CAD build for the part. Positions are in the model's coordinates, mm. A direction names the side the tool comes from. Give positions to 0.01 mm unless a question says otherwise; leave off trailing zeros. Order: outer loops, then holes, each group sorted by start corner. A loop starts at its lowest first (then second) coordinate and runs counter-clockwise, first axis right, second up. Notation, with made-up numbers: M 35.5,83.5 L 68.5,83.5 A20 ccw 68.5,103.5 Z; hole C 28,85 d9. An arc over 180 degrees is marked long. Put each result on its own line as item: value. Start each with the question number.
1) Tool access for faces 1 (the face through (0, 0, -10)), 2 (the face through (-40, 0, -20.629)): list every direction of +Z, -Z, +X, -X, +Y, -Y with a clear straight run to the whole face (end or side of a thin tool).
2) Cut at C-C (x = -42). Write the cut outline in (y, z).
3) Drill centre lines: line 1 (X direction, y = 0.85, z = -14.25); line 2 (Z direction, x = -44, y = 0.3); line 3 (Z direction, x = -44, y = 0.65). Where is each one in solid material? Low to high. Write a range as [from, to].
4) Cut at D-D (y = 0.35). Write the cut outline in (x, z), and give its area (3 significant figures).
5) Cut at A-A (z = -16). Write the cut outline in (x, y).
6) Cut at B-B (x = -6). Write the cut outline in (y, z), and give its area (3 significant figures).
7) Pin check, flat tips, straight feed: pin 1 (0.9 mm diameter, centred on x = -11.5, y = -0.5, fed in from -Z); pin 2 (0.9 mm diameter, centred on x = -40.5, y = 0.5, fed in from -Z); pin 3 (1.5 mm diameter, centred on x = -22, y = 1, fed in from -Z). Stop position of each tip, or through.
8) Two-plate mould, pull along Z, no slides. Class faces 3 (the face through (-25, 1.944, -6)), 4 (the face through (-45.5, 0.4, -2.2)), 5 (the face through (-15.406, 0, -14)), 6 (the face through (-24.65, 0.42, -23.37)): released by +Z, released by -Z, zero draft, split by the parting line, or undercut.
Autodesk Inventor part; units mm, degrees
ref_plane "YZ Plane" through (0, 0, 0) normal (1, 0, 0) x (0, 1, 0)
ref_plane "XZ Plane" through (0, 0, 0) normal (0, 1, 0) x (-1, 0, 0)
ref_plane "XY Plane" through (0, 0, 0) normal (0, 0, 1) x (1, 0, 0)
sketch "Sketch1" plane through (0, 0, 0) normal (1, 0, 0) x (0, 1, 0)
  line L0 (1.944, 4.8709) -> (-1.056, 4.8709)
  line L1 (-1.056, 4.8709) -> (-1.056, -25.1291)
  line L2 (-1.056, -25.1291) -> (1.944, -25.1291)
  line L3 (1.944, -25.1291) -> (1.944, 4.8709)
  line L4 (-1.056, -25.1291) -> (9.6963, -12.315)
  point P0 (0, 0)
  point P1 (1.944, -21.5539)
  dimension "d0" = 3
  dimension "d1" = 30
  dimension "d2" = 40
extrude "Extrusion1" add sketch "Sketch1" against normal blind 50 contours L3 L4 L1 L0
sketch "Szkic2" plane through (0, -1.056, -25.1291) normal (0, -1, 0) x (1, 0, 0)
  line L0 (0, 30) -> (0, 0)
  line L1 (0, 30) -> (-50, 30)
  line L2 (-50, 0) -> (-50, 30)
  line L3 (0, 0) -> (-50, 0)
  line L4 (-35.094, 16.557) -> (-35.094, 5.254)
  line L5 (-45, 5) -> (-35.348, 5)
  line L6 (-45, 5) -> (-45, 16.43)
  line L7 (-44.873, 16.557) -> (-35.094, 16.557)
  circle A0 centre (-39.92, 11.35) radius 1
  line L8 (-25, 0) -> (-25, 30)
  line L9 (-35.094, 5.254) -> (-35.348, 5)
  line L10 (-45.5, 16.43) -> (-45.5, 4.5)
  line L11 (-45.5, 4.5) -> (-35.1409, 4.5)
  line L12 (-34.594, 5.0469) -> (-34.594, 17.057)
  line L13 (-34.594, 17.057) -> (-44.873, 17.057)
  line L14 (-35.1409, 4.5) -> (-35.094, 4.5469)
  line L15 (-34.6409, 5) -> (-34.594, 5.0469)
  line L16 (-45.5, 4.5) -> (-34.594, 4.5)
  line L17 (-34.594, 4.5) -> (-34.594, 17.057)
  line L18 (-34.594, 17.057) -> (-45.5, 17.057)
  line L19 (-45.5, 17.057) -> (-45.5, 4.5)
  circle A1 centre (-10.08, 11.35) radius 1
  line L20 (-4.5, 16.43) -> (-4.5, 4.5)
  line L21 (-4.5, 4.5) -> (-14.8591, 4.5)
  line L22 (-15.406, 5.0469) -> (-15.406, 17.057)
  line L23 (-15.406, 17.057) -> (-5.127, 17.057)
  line L24 (-4.5, 4.5) -> (-15.406, 4.5)
  line L25 (-15.406, 4.5) -> (-15.406, 17.057)
  line L26 (-15.406, 17.057) -> (-4.5, 17.057)
  line L27 (-4.5, 17.057) -> (-4.5, 4.5)
  line L28 (0, 4.1492) -> (-50, 4.1492)
  line L29 (-50, 4.1492) -> (-50, 27.66)
  line L30 (-36.5, 27.66) -> (-50, 27.66)
  line L31 (-36.5, 27.66) -> (-36.5, 17.057)
  line L32 (-26.5, 4.66) -> (-36.5, 4.66)
  line L33 (-26.5, 4.66) -> (-26.5, 34.4086)
  line L34 (-23.5, 34.4086) -> (-23.5, 4.66)
  line L35 (-13.5, 4.66) -> (-23.5, 4.66)
  line L36 (-13.5, 4.66) -> (-13.5, 13.5389)
  line L37 (0, 27.66) -> (-13.5, 27.66)
  line L38 (0, 4.1492) -> (0, 27.66)
  line L39 (-50, 4.1492) -> (-44, 4.1492)
  line L40 (-44, 27.66) -> (-50, 27.66)
  line L41 (-50, 27.66) -> (-50, 4.1492)
  line L42 (-50, 27.66) -> (-36.5, 27.66)
  line L43 (-36.5, 27.66) -> (-36.5, 24.66)
  line L44 (-50, 24.66) -> (-50, 27.66)
  circle A2 centre (-10.08, 11.35) radius 1
  circle A3 centre (-39.92, 11.35) radius 1
  line L45 (-6, 27.66) -> (-6, 22.91)
  line L46 (-44, 27.66) -> (-44, 22.91)
  circle A4 centre (-6, 22.91) radius 1.5
  circle A5 centre (-44, 22.91) radius 1.5
  circle A6 centre (-6, 22.91) radius 1.75
  circle A7 centre (-44, 22.91) radius 1.75
  line L47 (-12.975, 17.057) -> (-13.5, 17.057)
  line L48 (-36.5, 17.057) -> (-37.0252, 17.057)
  line L49 (-45.5, 15.557) -> (-45.5, 15.0389)
  line L50 (-37.0252, 13.5389) -> (-36.5, 13.5389)
  line L51 (-36.5, 13.5389) -> (-36.5, 4.66)
  line L52 (-13.5, 13.5389) -> (-12.975, 13.5389)
  line L53 (-4.5, 15.0389) -> (-4.5, 15.557)
  arc A8 (-12, 17.057) -> (-12.975, 16.6969) centre (-12, 15.557) ccw
  line L54 (-12.975, 16.6969) -> (-12.975, 17.057)
  line L55 (-37.0252, 16.697) -> (-37.0252, 17.057)
  arc A9 (-37.0252, 16.697) -> (-38, 17.057) centre (-38, 15.557) ccw
  arc A10 (-44, 17.057) -> (-45.5, 15.557) centre (-44, 15.557) ccw
  arc A11 (-45.5, 15.0389) -> (-44, 13.5389) centre (-44, 15.0389) ccw
  arc A12 (-38, 13.5389) -> (-37.0252, 13.8988) centre (-38, 15.0389) ccw
  line L56 (-37.0252, 13.8988) -> (-37.0252, 13.5389)
  line L57 (-12.975, 13.899) -> (-12.975, 13.5389)
  arc A13 (-12.975, 13.899) -> (-12, 13.5389) centre (-12, 15.0389) ccw
  line L58 (-12, 13.5389) -> (-6, 13.5389)
  arc A14 (-6, 13.5389) -> (-4.5, 15.0389) centre (-6, 15.0389) ccw
  arc A15 (-4.5, 15.557) -> (-6, 17.057) centre (-6, 15.557) ccw
  line L59 (-6, 17.057) -> (-12, 17.057)
  line L60 (-38, 17.057) -> (-44, 17.057)
  line L61 (-44, 13.5389) -> (-38, 13.5389)
  arc A16 (-26.5, 34.4086) -> (-23.5, 34.4086) centre (-25, 35.31) ccw
  line L62 (-13.5, 17.057) -> (-13.5, 27.66)
  point P0 (0, 25.1291)
  point P1 (-45.5, 13.5389)
  point P2 (-4.5, 13.5389)
extrude "Wyciągnięcie proste2" cut sketch "Szkic2" against normal through all contours L35 L36 L52 L57 A13 L58 A14 L20 L21 L24 L25 | L25 L22 L23 L54 A8 A15 L20 A14 L58 A13 L57 L52 L36 L35 | L23 A8 L54 | L32 L51 L50 L56 A12 L61 A11 L10 A10 L13 A9 L55 L12 L17 | L17 L16 L11 L10 A11 L6 L5 L51 L32 | L23 L26 L27 L20 A15 | L5 L6 A11 L61 A12 L56 L50 L51 | L55 A9 L13 | L10 L19 L18 L13 A10 | A0 | A1
sketch "Szkic3" plane through (0, -1.056, -25.1291) normal (0, -1, 0) x (1, 0, 0)
  line L0 (-4.5, 17.057) -> (-4.5, 4.5)
  line L1 (-4.5, 4.5) -> (-15.406, 4.5)
  line L2 (-15.406, 4.5) -> (-15.406, 17.057)
  line L3 (-15.406, 17.057) -> (-4.5, 17.057)
  line L4 (-34.594, 17.057) -> (-34.594, 4.5)
  line L5 (-34.594, 4.5) -> (-45.5, 4.5)
  line L6 (-45.5, 4.5) -> (-45.5, 17.057)
  line L7 (-45.5, 17.057) -> (-34.594, 17.057)
  line L8 (0, 30) -> (0, 0)
  line L9 (0, 30) -> (-50, 30)
  line L10 (-50, 0) -> (-50, 30)
  line L11 (0, 0) -> (-50, 0)
  circle A0 centre (-44, 24.66) radius 1.75
  circle A1 centre (-10.08, 11.35) radius 1
  circle A2 centre (-39.92, 11.35) radius 1
  line L12 (0, 4.1492) -> (-50, 4.1492)
  line L13 (-50, 4.1492) -> (-50, 27.66)
  line L14 (-36.5, 27.66) -> (-50, 27.66)
  line L15 (-36.5, 27.66) -> (-36.5, 17.057)
  line L16 (-26.5, 4.66) -> (-36.5, 4.66)
  line L17 (-26.5, 4.66) -> (-26.5, 34.4086)
  line L18 (-23.5, 34.4086) -> (-23.5, 4.66)
  line L19 (-13.5, 4.66) -> (-23.5, 4.66)
  line L20 (-13.5, 4.66) -> (-13.5, 13.5389)
  line L21 (0, 27.66) -> (-13.5, 27.66)
  line L22 (0, 4.1492) -> (0, 27.66)
  line L23 (-44, 27.66) -> (-44, 22.91)
  line L24 (-6, 27.66) -> (-6, 22.91)
  circle A3 centre (-44, 22.91) radius 1.5
  circle A4 centre (-6, 22.91) radius 1.5
  circle A5 centre (-6, 22.91) radius 1.75
  circle A6 centre (-44, 22.91) radius 1.75
  line L25 (-12.975, 17.057) -> (-13.5, 17.057)
  line L26 (-36.5, 17.057) -> (-37.0252, 17.057)
  line L27 (-45.5, 15.557) -> (-45.5, 15.0389)
  line L28 (-37.0252, 13.5389) -> (-36.5, 13.5389)
  line L29 (-36.5, 13.5389) -> (-36.5, 4.66)
  line L30 (-13.5, 13.5389) -> (-12.975, 13.5389)
  line L31 (-4.5, 15.0389) -> (-4.5, 15.557)
  arc A7 (-12, 17.057) -> (-12.975, 16.6969) centre (-12, 15.557) ccw
  line L32 (-12.975, 16.6969) -> (-12.975, 17.057)
  line L33 (-37.0252, 16.697) -> (-37.0252, 17.057)
  arc A8 (-37.0252, 16.697) -> (-38, 17.057) centre (-38, 15.557) ccw
  arc A9 (-44, 17.057) -> (-45.5, 15.557) centre (-44, 15.557) ccw
  arc A10 (-45.5, 15.0389) -> (-44, 13.5389) centre (-44, 15.0389) ccw
  arc A11 (-38, 13.5389) -> (-37.0252, 13.8988) centre (-38, 15.0389) ccw
  line L34 (-37.0252, 13.8988) -> (-37.0252, 13.5389)
  line L35 (-12.975, 13.899) -> (-12.975, 13.5389)
  arc A12 (-12.975, 13.899) -> (-12, 13.5389) centre (-12, 15.0389) ccw
  line L36 (-12, 13.5389) -> (-6, 13.5389)
  arc A13 (-6, 13.5389) -> (-4.5, 15.0389) centre (-6, 15.0389) ccw
  arc A14 (-4.5, 15.557) -> (-6, 17.057) centre (-6, 15.557) ccw
  line L37 (-6, 17.057) -> (-12, 17.057)
  line L38 (-38, 17.057) -> (-44, 17.057)
  line L39 (-44, 13.5389) -> (-38, 13.5389)
  arc A15 (-26.5, 34.4086) -> (-23.5, 34.4086) centre (-25, 35.31) ccw
  line L40 (-13.5, 17.057) -> (-13.5, 27.66)
  point P0 (0, 25.1291)
  point P1 (-45.5, 13.5389)
  point P2 (-4.5, 13.5389)
  dimension "d13" = 3
  dimension "d14" = 3
extrude "Wyciągnięcie proste3" cut sketch "Szkic3" against normal through all contours A4 | A3 L23 A0 | A0 A3 | A3 A0 L23
properties part number "nozz" material "Stal nierdzewna"
Solution:
1. face 1: +Z, -Z, +X, +Y, -Y
1. face 2: +Y, -Y
2. outline: M -1.06,-25.13 L 1.94,-21.55 L 1.94,-20.63 L -1.06,-20.63 Z; M -1.06,-8.07 L 1.94,-8.07 L 1.94,4.87 L -1.06,4.87 Z
3. line 1: [-50, -45.5], [-34.59, -15.41], [-4.5, 0]
3. line 2: [-23.51, -20.63], [-8.07, -3.72], [-0.72, 4.87]
3. line 3: [-23.1, -20.63], [-8.07, -3.72], [-0.72, 4.87]
4. outline: M -50,-23.45 L 0,-23.45 L 0,4.87 L -50,4.87 Z; hole M -45.5,-20.63 L -34.59,-20.63 L -34.59,-8.07 L -45.5,-8.07 Z; hole C -44,-2.22 d3; hole M -15.41,-20.63 L -4.5,-20.63 L -4.5,-8.07 L -15.41,-8.07 Z; hole C -6,-2.22 d3
4. area: 1,130 mm²
5. outline: M -50,-1.06 L -45.5,-1.06 L -45.5,1.94 L -50,1.94 Z; M -34.59,-1.06 L -15.41,-1.06 L -15.41,1.94 L -34.59,1.94 Z; M -4.5,-1.06 L 0,-1.06 L 0,1.94 L -4.5,1.94 Z
6. outline: M -1.06,-25.13 L 1.94,-21.55 L 1.94,-20.63 L -1.06,-20.63 Z; M -1.06,-8.07 L 1.94,-8.07 L 1.94,-3.72 L -1.06,-3.72 Z; M -1.06,-0.72 L 1.94,-0.72 L 1.94,4.87 L -1.06,4.87 Z
6. area: 38.0 mm²
7. pin 1: z = -25
7. pin 2: z = -23.81
7. pin 3: z = -23.57
8. face 3: zero draft
8. face 4: undercut
8. face 5: undercut
8. face 6: released by -Z
